from build123d import *

# Parameters (mm, degrees)
CROQUIS2_W              = 22
CROQUIS2_H              = 11
SALIENTE_EXTRUIR1_DEPTH = 11
CROQUIS4_W              = 13
CROQUIS4_H              = 3.3
CROQUIS4_W_2            = 11
CROQUIS4_H_2            = 3
SALIENTE_EXTRUIR2_DEPTH = 11
REDONDEO1_RADIUS        = 5.5
REDONDEO1_LENGTH        = 3
REDONDEO2_RADIUS        = 5.5
REDONDEO2_LENGTH        = 3.3
REDONDEO3_RADIUS        = 5.5
REDONDEO3_LENGTH        = 3.3
CROQUIS7_R              = 1.6
CORTAR_EXTRUIR3_DEPTH   = 27.428025294
CROQUIS8_R              = 1.6
CORTAR_EXTRUIR4_DEPTH   = 28.575134105


with BuildPart() as part:
    # Croquis2 → Saliente-Extruir1 (new body)
    with BuildSketch(Plane.XY):
        with Locations((-0.996999741, -40.458999634)):
            Rectangle(CROQUIS2_W, CROQUIS2_H)
    extrude(amount=SALIENTE_EXTRUIR1_DEPTH)

    # Croquis4 → Saliente-Extruir2 (add)
    with BuildSketch(Plane.XY.offset(11)):
        with Locations((16.503000259, -43.808999634)):
            Rectangle(CROQUIS4_W, CROQUIS4_H)
        with Locations((-17.496999741, -40.508999634)):
            Rectangle(CROQUIS4_W_2, CROQUIS4_H_2)
        with Locations((16.503000259, -37.108999634)):
            Rectangle(CROQUIS4_W, CROQUIS4_H)
    extrude(amount=-SALIENTE_EXTRUIR2_DEPTH)

    # Redondeo1: full round fillet: the end face becomes a half cylinder, R = half its width
    redondeo1_face = Plane((-22.996999741, -40.508999634, 5.5), x_dir=(0, -1, 0), z_dir=(-1, 0, 0))  # on the end face: x along it, z out of the body
    redondeo1_slab = redondeo1_face.offset(-REDONDEO1_RADIUS / 2) * Box(REDONDEO1_LENGTH, 2 * REDONDEO1_RADIUS, REDONDEO1_RADIUS, mode=Mode.PRIVATE)  # the body's end, R deep
    redondeo1_round = Plane((-17.496999741, -40.508999634, 5.5), x_dir=(-1, 0, 0), z_dir=(0, -1, 0)) * Cylinder(REDONDEO1_RADIUS, REDONDEO1_LENGTH, mode=Mode.PRIVATE)  # its axis R under the face
    add(redondeo1_slab - redondeo1_round, mode=Mode.SUBTRACT)

    # Redondeo2: full round fillet: the end face becomes a half cylinder, R = half its width
    redondeo2_face = Plane((23.003000259, -37.108999634, 5.5), x_dir=(0, 1, 0), z_dir=(1, 0, 0))  # on the end face: x along it, z out of the body
    redondeo2_slab = redondeo2_face.offset(-REDONDEO2_RADIUS / 2) * Box(REDONDEO2_LENGTH, 2 * REDONDEO2_RADIUS, REDONDEO2_RADIUS, mode=Mode.PRIVATE)  # the body's end, R deep
    redondeo2_round = Plane((17.503000259, -37.108999634, 5.5), x_dir=(1, 0, 0), z_dir=(0, 1, 0)) * Cylinder(REDONDEO2_RADIUS, REDONDEO2_LENGTH, mode=Mode.PRIVATE)  # its axis R under the face
    add(redondeo2_slab - redondeo2_round, mode=Mode.SUBTRACT)

    # Redondeo3: full round fillet: the end face becomes a half cylinder, R = half its width
    redondeo3_face = Plane((23.003000259, -43.808999634, 5.5), x_dir=(0, 1, 0), z_dir=(1, 0, 0))  # on the end face: x along it, z out of the body
    redondeo3_slab = redondeo3_face.offset(-REDONDEO3_RADIUS / 2) * Box(REDONDEO3_LENGTH, 2 * REDONDEO3_RADIUS, REDONDEO3_RADIUS, mode=Mode.PRIVATE)  # the body's end, R deep
    redondeo3_round = Plane((17.503000259, -43.808999634, 5.5), x_dir=(1, 0, 0), z_dir=(0, 1, 0)) * Cylinder(REDONDEO3_RADIUS, REDONDEO3_LENGTH, mode=Mode.PRIVATE)  # its axis R under the face
    add(redondeo3_slab - redondeo3_round, mode=Mode.SUBTRACT)

    # Croquis7 → Cortar-Extruir3 (cut, through all)
    with BuildSketch(Plane(origin=(0, -39.008999634, 0), x_dir=(1, 0, 0), z_dir=(0, 1, 0))):
        with Locations(Location((-17.496999741, -5.5, 0), (0, 0, 270))):
            Circle(CROQUIS7_R)
    extrude(amount=-CORTAR_EXTRUIR3_DEPTH, mode=Mode.SUBTRACT)

    # Croquis8 → Cortar-Extruir4 (cut, through all)
    with BuildSketch(Plane(origin=(0, -35.458999634, 0), x_dir=(1, 0, 0), z_dir=(0, 1, 0))):
        with Locations(Location((17.503000259, -5.5, 0), (0, 0, 270))):
            Circle(CROQUIS8_R)
    extrude(amount=-CORTAR_EXTRUIR4_DEPTH, mode=Mode.SUBTRACT)


solid = part.part
Work out the finished part from the listing and answer in its coordinate system (mm). A direction names the side the tool comes from. Round coordinates to 2 decimals unless told otherwise and drop trailing zeros. Loops run counter-clockwise (first coordinate to the right, second up) from the corner with the lowest first, then second, coordinate; pieces in that order, holes last. Notation, with made-up numbers: M -7.5,23.5 L 18.5,23.5 A30 ccw 18.5,53.5 Z; hole C -27.5,71 d10. An arc over 180 degrees is marked long. One line per question, with ' | ' between items. Start each with the question number.
(1) A cutting plane is placed at B-B on z = 5.5. Write down the section's boundary in (x, y).
(2) A cutting plane is placed at D-D on x = 18.5. Write down the section's boundary in (y, z).
(3) A cutting plane is placed at C-C on y = -43.25. Write down the section's boundary in (x, z), plus the area to 3 significant figures.
(4) A cutting plane is placed at A-A on x = 13.5. Write down the section's boundary in (y, z), plus the area to 3 significant figures.
(5) Flat-ended cylindrical pins translate along their axes: pin 1 Ø1 at (y, z) = (-44.5, 3.5) entering from +X; pin 2 Ø3.5 at (x, z) = (18, 8) entering from -Y; pin 3 Ø1.5 at (x, z) = (-16, 8.5) entering from -Y. Find the tip coordinate at first contact, or state that the pin passes through.
(6) For a pull along Y with two mould halves and no side action, classify faces 4 (the face through (15, -42.159, 6)), 5 (the face through (23, -37.09, 5.62)), 6 (the face through (-1, -45.959, 5)) as released by +Y, released by -Y, zero draft, split by the parting line, or undercut.
(7) A tool of negligible diameter and unlimited length cuts with its end or side. For faces 1 (the face through (15, -45.459, 6)), 2 (the face through (-16, -39.009, 4)), 3 (the face through (10.003, -40, 5)), from which of +Z, -Z, +X, -X, +Y, -Y can it reach the whole face along a straight path? Write none if from no direction.
(8) Find the intervals of material crossed by line 1 (X direction, y = -40.7, z = 5.5); line 2 (X direction, y = -36.75, z = 5.5); line 3 (Y direction, x = 11.5, z = 9.5), in increasing order.
Geometry check:
1) outline: M -23,-42.01 L -19.1,-42.01 L -19.1,-39.01 L -23,-39.01 Z; M -15.9,-42.01 L -12,-42.01 L -12,-45.96 L 10,-45.96 L 10,-45.46 L 15.9,-45.46 L 15.9,-42.16 L 10,-42.16 L 10,-38.76 L 15.9,-38.76 L 15.9,-35.46 L 10,-35.46 L 10,-34.96 L -12,-34.96 L -12,-39.01 L -15.9,-39.01 Z; M 19.1,-45.46 L 23,-45.46 L 23,-42.16 L 19.1,-42.16 Z; M 19.1,-38.76 L 23,-38.76 L 23,-35.46 L 19.1,-35.46 Z
2) outline: M -45.46,0.09 L -42.16,0.09 L -42.16,4.25 L -45.46,4.25 Z; M -45.46,6.75 L -42.16,6.75 L -42.16,10.91 L -45.46,10.91 Z; M -38.76,0.09 L -35.46,0.09 L -35.46,4.25 L -38.76,4.25 Z; M -38.76,6.75 L -35.46,6.75 L -35.46,10.91 L -38.76,10.91 Z
3) outline: M -12,0 L 17.5,0 A5.5 ccw 17.5,11 L -12,11 Z; hole C 17.5,5.5 d3.2 | area: 364 mm²
4) outline: M -45.46,0 L -42.16,0 L -42.16,11 L -45.46,11 Z; M -38.76,0 L -35.46,0 L -35.46,11 L -38.76,11 Z | area: 72.6 mm²
5) pin 1: stops at x = 22.79 | pin 2: stops at y = -45.46 | pin 3: stops at y = -42.01
6) face 4: undercut | face 5: zero draft | face 6: released by -Y
7) face 1: +Z, -Z, +X, -Y | face 2: +Z, -Z, -X, +Y | face 3: +Z, -Z, +X
8) line 1: x = -23 to -19.1, -15.9 to 10 | line 2: x = -12 to 15.9, 19.1 to 23 | line 3: y = -45.46 to -42.16, -38.76 to -35.46
